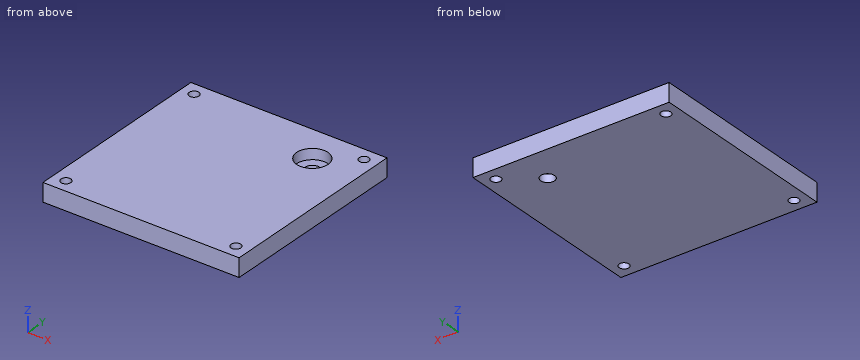
```python
from build123d import *

# Parameters (mm, degrees)
SKETCH1_W           = 95.25
SKETCH1_H           = 95.25
BOSS_EXTRUDE1_DEPTH = 8.89
SKETCH2_OUTSIDE_W   = 124.25
SKETCH2_OUTSIDE_H   = 124.25
SKETCH2_OUTSIDE_W_2 = 95.25
SKETCH2_OUTSIDE_H_2 = 95.25
SKETCH2_OUTSIDE_R   = 2.38125
CUT_EXTRUDE2_DEPTH  = 9.89
SKETCH3_R           = 7.62
CUT_EXTRUDE3_DEPTH  = 5.08
SKETCH4_R           = 3.3655
CUT_EXTRUDE4_DEPTH  = 4.81


with BuildPart() as part:
    # Sketch1 → Boss-Extrude1 (new body)
    with BuildSketch(Plane.XY):
        Rectangle(SKETCH1_W, SKETCH1_H)
    extrude(amount=BOSS_EXTRUDE1_DEPTH)

    # Sketch2 outside → Cut-Extrude2 (cut, through all)
    with BuildSketch(Plane.XY.offset(8.89)):
        Rectangle(SKETCH2_OUTSIDE_W, SKETCH2_OUTSIDE_H)
        Rectangle(SKETCH2_OUTSIDE_W_2, SKETCH2_OUTSIDE_H_2, mode=Mode.SUBTRACT)
        with Locations((-41.275, 41.275)):
            Circle(SKETCH2_OUTSIDE_R)
        with Locations((41.275, 41.275)):
            Circle(SKETCH2_OUTSIDE_R)
        with Locations((41.275, -41.275)):
            Circle(SKETCH2_OUTSIDE_R)
        with Locations((-41.275, -41.275)):
            Circle(SKETCH2_OUTSIDE_R)
    extrude(amount=-CUT_EXTRUDE2_DEPTH, mode=Mode.SUBTRACT)

    # Sketch3 → Cut-Extrude3 (cut)
    with BuildSketch(Plane.XY.offset(8.89)):
        with Locations((24.765, 29.845)):
            Circle(SKETCH3_R)
    extrude(amount=-CUT_EXTRUDE3_DEPTH, mode=Mode.SUBTRACT)

    # Sketch4 → Cut-Extrude4 (cut, through all)
    with BuildSketch(Plane.XY.offset(3.81)):
        with Locations((24.765, 29.845)):
            Circle(SKETCH4_R)
    extrude(amount=-CUT_EXTRUDE4_DEPTH, mode=Mode.SUBTRACT)


solid = part.part
```
Geometry check sheet. Reference: the model listing, model coordinates, mm. Give positions to 0.01 mm unless a question says otherwise; leave off trailing zeros. Write each loop counter-clockwise with the first axis right and the second up, starting at its lowest first coordinate (ties: lowest second). Pieces come first, ordered by that corner, then holes.
1) Section check A-A, the plane x = 26. Record the boundary of the cut face in (y, z) (3 decimals), and give its area (3 significant figures).
2) Gauge pin test, flat end, axial feed: pin 1 (7.5 mm diameter, centred on x = -41.275, y = -41.275, fed in from +Z). Record the tip position at first contact, or that the pin passes through.
3) Section check B-B, the plane z = 6.5. Record the boundary of the cut face in (x, y) (1 decimal), and give its area (3 significant figures).
4) Material ranges on L1, parallel to Y at x = 41.5, z = 6.25 (3 decimals); L2, parallel to X at y = -43, z = 3.75 (3 decimals); L3, parallel to X at y = -40, z = 4 (3 decimals), recorded low to high.
Computed:
1. outline: (-47.625, 0) - (26.714, 0) - (26.714, 3.81) - (22.326, 3.81) - (22.326, 8.89) - (-47.625, 8.89) - close; (32.976, 0) - (47.625, 0) - (47.625, 8.89) - (37.364, 8.89) - (37.364, 3.81) - (32.976, 3.81) - close
1. area: 747 mm2
2. pin 1: stops at z = 8.89
3. outline: (-47.6, -47.6) - (47.6, -47.6) - (47.6, 47.6) - (-47.6, 47.6) - close; hole circle Ø4.8 at (-41.3, -41.3); hole circle Ø4.8 at (-41.3, 41.3); hole circle Ø15.2 at (24.8, 29.8); hole circle Ø4.8 at (41.3, -41.3); hole circle Ø4.8 at (41.3, 41.3)
3. area: 8,820 mm2
4. L1: y = -47.625 to -43.646, -38.904 to 38.904, 43.646 to 47.625
4. L2: x = -47.625 to -42.917, -39.633 to 39.633, 42.917 to 47.625
4. L3: x = -47.625 to -43.286, -39.264 to 39.264, 43.286 to 47.625
